```python
from build123d import *

# Parameters (mm, degrees)
SKETCH1_W             = 25
SKETCH1_H             = 15
SKETCH1_R             = 4.5
SKETCH1_R_2           = 1.1303
BOSS_EXTRUDE1_DEPTH   = 6.35
F_4_40_TAPPED_HOLE1_D = 2.2606
FILLET1_R             = 2


with BuildPart() as part:
    # Sketch1 → Boss-Extrude1 (new body)
    with BuildSketch(Plane.XY):
        with Locations((12.5, -7.5)):
            Rectangle(SKETCH1_W, SKETCH1_H)
        with Locations((12.5, -7.5)):
            Circle(SKETCH1_R, mode=Mode.SUBTRACT)
        with Locations((3.5, -7.5)):
            Circle(SKETCH1_R_2, mode=Mode.SUBTRACT)
        with Locations((21.5, -7.5)):
            Circle(SKETCH1_R_2, mode=Mode.SUBTRACT)
    extrude(amount=BOSS_EXTRUDE1_DEPTH)

    # #4-40 Tapped Hole1 (through all)
    with Locations(Plane(origin=(21.5, -7.5, 6.35), x_dir=(1, 0, 0), z_dir=(0, 0, 1))):
        with Locations((0, 0), (-18, 0)):
            Hole(F_4_40_TAPPED_HOLE1_D / 2)

    # Fillet1
    fillet1_edges = [part.edges().sort_by_distance(p)[0] for p in [
        (0, 0, 3.175),
        (25, 0, 3.175),
        (25, -15, 3.175),
        (0, -15, 3.175),
    ]]
    fillet(fillet1_edges, radius=FILLET1_R)


solid = part.part
```
The model under review builds one solid part; all positions refer to its coordinate system, in mm. Round coordinates to 2 decimals unless told otherwise and drop trailing zeros. Loops run counter-clockwise (first coordinate to the right, second up) from the corner with the lowest first, then second, coordinate; pieces in that order, holes last.
1) Consider section B-B on z = 4.5. State the section outline as (x, y) points.
Values follow:
outline: (0, -13) arc R2 ccw to (2, -15) - (23, -15) arc R2 ccw to (25, -13) - (25, -2) arc R2 ccw to (23, 0) - (2, 0) arc R2 ccw to (0, -2) - close; hole circle Ø2.26 at (3.5, -7.5); hole circle Ø9 at (12.5, -7.5); hole circle Ø2.26 at (21.5, -7.5)
2) The part is to be moulded in two halves that separate along Y. For faces 1 (the face through (0.57, -0.6, 3.22)), 2 (the face through (25, -8, 3)), 3 (the face through (22.544, -7.933, 3.131)), say which applies: pulls with the +Y half, pulls with the -Y half, needs draft (parallel to the pull), parting line crosses it, or undercut.
Values follow:
face 1: pulls with the +Y half
face 2: needs draft
face 3: undercut
3) Consider section D-D on y = -11.25. State the section outline as (x, z) points.
Values follow:
outline: (0, 0) - (10.01, 0) - (10.01, 6.35) - (0, 6.35) - close; (14.99, 0) - (25, 0) - (25, 6.35) - (14.99, 6.35) - close
4) Wall thickness on line 1 along Y through (x, z) = (12.5, 2.25); line 2 along X through (y, z) = (-7.75, 5.5); line 3 along Y through (x, z) = (3.5, 2.5): over which ranges is each line inside the solid? List them lowest first.
Values follow:
line 1: y = -15 to -12, -3 to 0
line 2: x = 0 to 2.4, 4.6 to 8.01, 16.99 to 20.4, 22.6 to 25
line 3: y = -15 to -8.63, -6.37 to 0
5) Consider section C-C on y = -7.5. State the section outline as (x, z) points.
Values follow:
outline: (0, 0) - (2.37, 0) - (2.37, 6.35) - (0, 6.35) - close; (4.63, 0) - (8, 0) - (8, 6.35) - (4.63, 6.35) - close; (17, 0) - (20.37, 0) - (20.37, 6.35) - (17, 6.35) - close; (22.63, 0) - (25, 0) - (25, 6.35) - (22.63, 6.35) - close
6) Consider section A-A on x = 21.5. State the section outline as (y, z) points, then the cut area to 3 significant figures.
Values follow:
outline: (-15, 0) - (-8.63, 0) - (-8.63, 6.35) - (-15, 6.35) - close; (-6.37, 0) - (0, 0) - (0, 6.35) - (-6.37, 6.35) - close
area: 80.9 mm2
